Build history of the part. All positions in model axes, mm. Coordinates: 2 decimals unless noted, no trailing zeros.
(1) Flat gauge pins, fed straight in: P1, Ø3, axis at x = 7, z = 70.5, coming from the -Y side; P2, Ø10, axis at x = 1, z = 42, coming from the -Y side; P3, Ø10, axis at x = 48, z = 59.5, coming from the -Y side. Where does each tip first touch, or does it go through?
(2) Wall check: L1, parallel to Z at x = 20, y = -17; L2, parallel to Y at x = 26, z = 54; L3, parallel to Y at x = 22, z = 74.5. Give the ranges that are in metal, low to high.
(3) Two-plate mould, pull along Z, no slides. Class faces 1 (the face through (0, 0, 0)), 2 (the face through (35.2, -47.3, 100)), 3 (the face through (0, 0, 2.5)): pulls with the +Z half, pulls with the -Z half, needs draft (parallel to the pull), parting line crosses it, or undercut.
from build123d import *

# Parameters (mm, degrees)
F4_T = -2.5


with BuildPart() as f3:
    # F2 (on offset) → F3 section 0
    with BuildSketch(Plane.XY.offset(100)):
        Polygon((31.682645, 13.290587), (0, 0), (-4.331336, -34.083269), (23.019972, -54.875951), (54.702617, -41.585363), (59.033954, -7.502094), align=None)
    # F1 (on Top) → F3 section 1
    with BuildSketch(Plane.XY):
        Polygon((-27.569018, 18.579667), (-29.874973, -14.585637), (-2.305955, -33.165304), (27.569018, -18.579667), (29.874973, 14.585637), (2.305955, 33.165304), align=None)
    loft()

    # F4
    f4_openings = [f3.faces().sort_by_distance(p)[0] for p in [
        (27.351309, -20.792682, 100),
    ]]
    offset(amount=F4_T, openings=f4_openings)


solid = f3.part
Response values:
1. P1: stops at y = -43.29
1. P2: stops at y = -40.63
1. P3: stops at y = -33.19
2. L1: z = 0 to 2.5
2. L2: y = -38.3 to -35.43, 13.71 to 16.79
2. L3: y = -46.97 to -44.12, 14.56 to 17.4
3. face 1: pulls with the -Z half
3. face 2: pulls with the +Z half
3. face 3: undercut
